Design review of the part shown in the three views and the two pictorial views. Dimensions are in mm from the part's minimum x, y and z. Round coordinates to 2 decimals unless told otherwise and drop trailing zeros. Write each loop counter-clockwise with the first axis right and the second up, starting at its lowest first coordinate (ties: lowest second). Pieces come first, ordered by that corner, then holes. Notation, with made-up numbers: (73, -37) -> (115, -37) arc R28 ccw to (115, -11) -> close; hole circle Ø1 at (69.5, 10). An arc over 180 degrees is marked (long way). One line per question, with ' | ' between items. Start each with the question number.
1) Consider section A-A (y = 15). Give the boundary of the cut face in (x, z), then the cut area to 3 significant figures.
2) Insertion check: pin 1 Ø8.5 at (x, y) = (66.5, 15) entering from +Z; pin 2 Ø6.5 at (x, y) = (66.5, 15) entering from +Z. Each pin has a flat end and moves straight along its axis. Give the tip position at first contact, or say it passes through.
3) Consider section C-C (x = 37.5). Give the boundary of the cut face in (y, z).
4) Mouldability with a two-part tool opening along X and no side actions: class the marked faces 1, 2, 3 and 4 as +X half, -X half, draft (parallel to the pull), parting line (faces both ways), or undercut.
5) Consider section D-D (x = 8.5). Give the boundary of the cut face in (y, z).
6) Consider section B-B (z = 32.5). Give the boundary of the cut face in (x, y).
7) For probe 1 along Y at (x, z) = (66.5, 61.85); probe 2 along Y at (x, z) = (66.5, 20); probe 3 along Z at (x, y) = (37.5, 41), list the stretches that pass through material, from the lowest coordinate up.
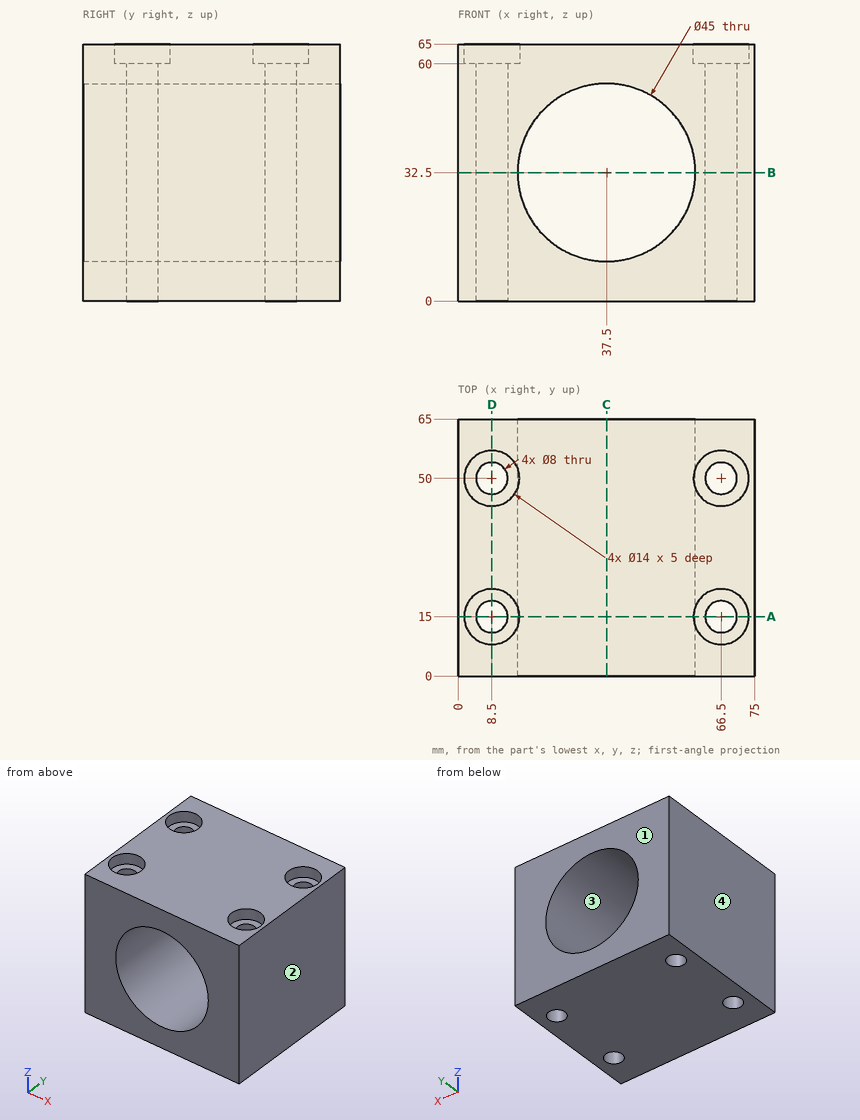
From the geometry:
1) outline: (0, 0) -> (4.5, 0) -> (4.5, 60) -> (1.5, 60) -> (1.5, 65) -> (0, 65) -> close; (12.5, 0) -> (62.5, 0) -> (62.5, 60) -> (59.5, 60) -> (59.5, 65) -> (15.5, 65) -> (15.5, 60) -> (12.5, 60) -> close; (70.5, 0) -> (75, 0) -> (75, 65) -> (73.5, 65) -> (73.5, 60) -> (70.5, 60) -> close; hole circle Ø45 at (37.5, 32.5) | area: 2,180 mm2
2) pin 1: stops at z = 60 | pin 2: passes through
3) outline: (0, 0) -> (65, 0) -> (65, 10) -> (0, 10) -> close; (0, 55) -> (65, 55) -> (65, 65) -> (0, 65) -> close
4) face 1: draft | face 2: +X half | face 3: undercut | face 4: -X half
5) outline: (0, 0) -> (11, 0) -> (11, 60) -> (8, 60) -> (8, 65) -> (0, 65) -> close; (19, 0) -> (46, 0) -> (46, 60) -> (43, 60) -> (43, 65) -> (22, 65) -> (22, 60) -> (19, 60) -> close; (54, 0) -> (65, 0) -> (65, 65) -> (57, 65) -> (57, 60) -> (54, 60) -> close
6) outline: (0, 0) -> (15, 0) -> (15, 65) -> (0, 65) -> close; (60, 0) -> (75, 0) -> (75, 65) -> (60, 65) -> close; hole circle Ø8 at (8.5, 15); hole circle Ø8 at (8.5, 50); hole circle Ø8 at (66.5, 15); hole circle Ø8 at (66.5, 50)
7) probe 1: y = 0 to 8, 22 to 43, 57 to 65 | probe 2: y = 0 to 11, 19 to 46, 54 to 65 | probe 3: z = 0 to 10, 55 to 65
